```python
from build123d import *

# Parameters (mm, degrees)
F0_W     = 152.4
F0_H     = 101.6
F0_R     = 38.1
F1_DEPTH = 19.05
F2_R     = 12.742658
F3_DEPTH = 25.4
F4_R     = 2.050488
F5_DEPTH = 25.4


with BuildPart() as f1:
    # F0 (on Front) → F1 (new body)
    with BuildSketch(Plane.XZ):
        with Locations((2.370438, -11.722004)):
            Rectangle(F0_W, F0_H)
        with Locations((33.632447, -16.140074)):
            Circle(F0_R, mode=Mode.SUBTRACT)
    extrude(amount=F1_DEPTH)

    # F2 (on face) → F3 (cut)
    with BuildSketch(Plane.XZ.offset(19.05)):
        with Locations((-41.844524, 14.192783)):
            Circle(F2_R)
    extrude(amount=-F3_DEPTH, mode=Mode.SUBTRACT)

    # F4 (on face) → F5 (cut)
    with BuildSketch(Plane.XZ.offset(19.05)):
        with Locations((9.855603, 18.817487)):
            Circle(F4_R)
        with Locations((-1.325114, -39.916918)):
            Circle(F4_R)
        with Locations((57.409292, -51.097635)):
            Circle(F4_R)
        with Locations((68.590008, 7.636771)):
            Circle(F4_R)
    extrude(amount=-F5_DEPTH, mode=Mode.SUBTRACT)


solid = f1.part
```
Input: part model. Units: mm. Frame: model coordinates. Coordinates: 2 decimals unless noted, no trailing zeros. Write each loop counter-clockwise with the first axis right and the second up, starting at its lowest first coordinate (ties: lowest second). Pieces come first, ordered by that corner, then holes. Notation, with made-up numbers: M -16.75,47 L 25.25,47 A20 ccw 25.25,82 Z; hole C 30,23 d3. An arc over 180 degrees is marked long. Use one line per item in the form item = value.
Q1. Draft query along Z for faces 1 (the face through (1, -9, -62.522)), 2 (the face through (-16, 0, -11)), 3 (the face through (-29.69, -9.66, 18.02)), 4 (the face through (1, -9, 39.078)). Return one class per face: released by +Z, released by -Z, zero draft, split by the parting line, or undercut.
Answer below:
face_1 = released by -Z
face_2 = zero draft
face_3 = undercut
face_4 = released by +Z
Q2. Section A-A (x = 30). Return loops of the section in (y, z).
Answer below:
outline = M -19.05,-62.52 L 0,-62.52 L 0,-54.07 L -19.05,-54.07 Z; M -19.05,21.79 L 0,21.79 L 0,39.08 L -19.05,39.08 Z
Q3. Section C-C (y = -5). Return loops of the section in (x, z), plus the area to 3 significant figures.
Answer below:
outline = M -73.83,-62.52 L 78.57,-62.52 L 78.57,39.08 L -73.83,39.08 Z; hole C -41.84,14.19 d25.49; hole C 33.63,-16.14 d76.2; hole C -1.33,-39.92 d4.1; hole C 9.86,18.82 d4.1; hole C 57.41,-51.1 d4.1; hole C 68.59,7.64 d4.1
area = 10,400 mm²
Q4. Section B-B (z = -25). Return loops of the section in (x, y).
Answer below:
outline = M -73.83,-19.05 L -3.42,-19.05 L -3.42,0 L -73.83,0 Z; M 70.69,-19.05 L 78.57,-19.05 L 78.57,0 L 70.69,0 Z
Q5. First-contact query: pin 1 (3.5 mm diameter, centred on x = -1.33, z = -39.92, fed in from -Y). Flat tip, straight axial feed; report the tip coordinate or a pass-through.
Answer below:
pin_1 = through
Q6. Material intervals for probe 1 along Z at (x, y) = (10, -12) (3 decimals); probe 2 along X at (y, z) = (-13.5, -7); probe 3 along X at (y, z) = (-10.5, 3), sorted ascending. Write a range as from..to.
Answer below:
probe_1 = -62.522..-46.025, 13.745..16.772, 20.863..39.078
probe_2 = -73.83..-3.35, 70.62..78.57
probe_3 = -73.83..-47.94, -35.75..0.69, 66.58..78.57
